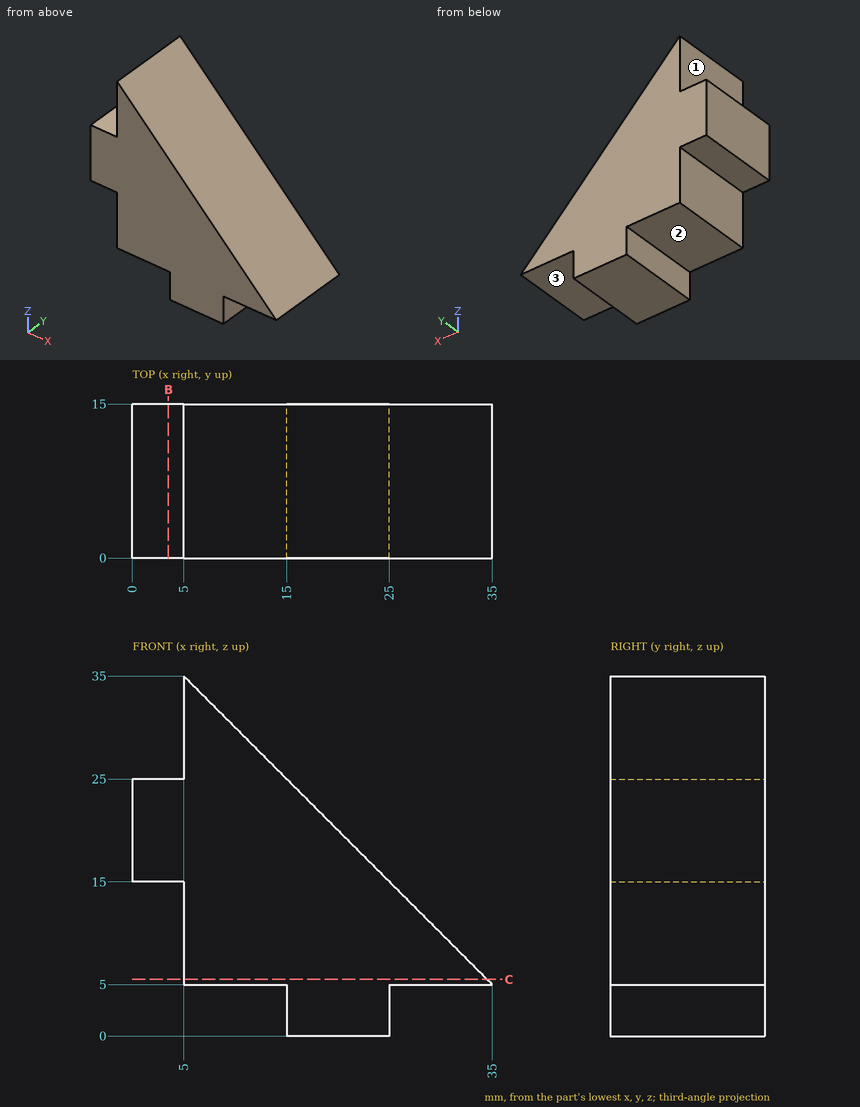
Can you work these out from the drawing? Everything is in mm from the part's minimum corner. A direction names the side the tool comes from. Coordinates: 2 decimals unless noted, no trailing zeros. Loops run counter-clockwise (first coordinate to the right, second up) from the corner with the lowest first, then second, coordinate; pieces in that order, holes last.
1. For the marked faces 1, 2 and 3, which set-ups out of +Z, -Z, +X, -X, +Y, -Y let a thin tool reach every point of the face, with its end or its side?
2. Imagine slicing it at C-C, the plane z = 5.5. Please give me the cut outline in (x, y), and give its area (4 significant figures).
3. For P1, Ø2.5, axis at y = 10.5, z = 3, coming from the -X side; P2, Ø1, axis at y = 8, z = 31.5, coming from the -X side; P3, Ø1, axis at x = 10, y = 10, coming from the +Z side, each with a flat end and sliding along its axis, tell me the tip position at first contact or that it passes through.
4. I need wall thicknesses on L1, parallel to Z at x = 4, y = 12.25; L2, parallel to Z at x = 14, y = 4.5; L3, parallel to X at y = 6.75, z = 26. Which ranges of each line are inside material? Lowest first, please.
5. Imagine slicing it at B-B, the plane x = 3.5. Please give me the cut outline in (y, z).
Taken from the geometry:
1. face 1: +Z, -X, +Y, -Y
1. face 2: -Z, -X, +Y, -Y
1. face 3: -Z, +X, +Y, -Y
2. outline: (5, 0) - (34.5, 0) - (34.5, 15) - (5, 15) - close
2. area: 442.5 mm2
3. P1: stops at x = 15
3. P2: stops at x = 5
3. P3: stops at z = 30.5
4. L1: z = 15 to 25
4. L2: z = 5 to 26
4. L3: x = 5 to 14
5. outline: (0, 15) - (15, 15) - (15, 25) - (0, 25) - close
